```python
from build123d import *

# Parameters (mm, degrees)
F1_DEPTH = 4.4


with BuildPart() as f1:
    # F0 (on Top) → F1 (new body)
    with BuildSketch(Plane.XY):
        with BuildLine():
            ThreePointArc((-12.44334, -91.95904), (-8.617964, -88.425467), (-3.570689, -87.143026))
            Line((-3.570689, -87.143026), (-3.570689, -70.3213))
            Line((-3.570689, -70.3213), (-82.913134, -70.3213))
            Line((-82.913134, -70.3213), (-88.507661, -70.3213))
            Line((-88.507661, -70.3213), (-88.507661, -75.559488))
            Line((-88.507661, -75.559488), (-84.057661, -75.559488))
            Line((-84.057661, -75.559488), (-84.057661, -80.009488))
            Line((-84.057661, -80.009488), (-88.507661, -80.009488))
            Line((-88.507661, -80.009488), (-88.507661, -96.734692))
            ThreePointArc((-88.507661, -96.734692), (-79.443295, -109.014634), (-64.98152, -113.89488))
            Line((-64.98152, -113.89488), (-45.348551, -113.89488))
            ThreePointArc((-45.348551, -113.89488), (-25.575249, -107.908225), (-12.44334, -91.95904))
        make_face()
        with BuildLine():
            ThreePointArc((-78.507661, -78.3213), (-77.628981, -76.199979), (-75.507661, -75.3213))
            Line((-75.507661, -75.3213), (-8.347679, -75.3213))
            ThreePointArc((-8.347679, -75.3213), (-6.986534, -76.530687), (-6.480797, -78.279848))
            Line((-6.480797, -78.279848), (-6.480797, -81.040353))
            Line((-6.480797, -81.040353), (-6.480797, -81.041593))
            ThreePointArc((-6.480797, -81.041593), (-7.309408, -82.599272), (-8.960268, -83.221863))
            ThreePointArc((-8.960268, -83.221863), (-13.595876, -85.631372), (-16.90926, -89.67069))
            ThreePointArc((-16.90926, -89.67069), (-28.184907, -103.637987), (-45.348551, -108.89488))
            Line((-45.348551, -108.89488), (-64.926874, -108.89488))
            ThreePointArc((-64.926874, -108.89488), (-76.195022, -105.191008), (-83.507661, -95.852104))
            Line((-83.507661, -95.852104), (-83.507661, -87.279848))
            ThreePointArc((-83.507661, -87.279848), (-82.921875, -85.865634), (-81.507661, -85.279848))
            ThreePointArc((-81.507661, -85.279848), (-79.386341, -84.401168), (-78.507661, -82.279848))
            Line((-78.507661, -82.279848), (-78.507661, -78.3213))
        make_face(mode=Mode.SUBTRACT)
        with BuildLine():
            Line((80.823653, -96.734275), (80.823653, -85.451687))
            Line((80.823653, -85.451687), (80.823653, -80.451687))
            Line((80.823653, -80.451687), (76.373653, -80.449196))
            Line((76.373653, -80.449196), (76.376145, -75.999196))
            Line((76.376145, -75.999196), (80.823653, -76.001686))
            Line((80.823653, -76.001686), (80.823653, -75.281577))
            Line((80.823653, -75.281577), (80.823653, -70.3213))
            Line((80.823653, -70.3213), (76.384345, -70.3213))
            Line((76.384345, -70.3213), (75.771756, -70.3213))
            Line((75.771756, -70.3213), (-3.570689, -70.3213))
            Line((-3.570689, -70.3213), (-3.570689, -87.143026))
            ThreePointArc((-3.570689, -87.143026), (1.080367, -88.217483), (4.786777, -91.225688))
            ThreePointArc((4.786777, -91.225688), (5.069545, -91.596309), (5.335725, -91.979017))
            ThreePointArc((5.335725, -91.979017), (18.457726, -107.907175), (38.207173, -113.894871))
            ThreePointArc((38.207173, -113.894871), (38.219889, -113.894877), (38.232605, -113.89488))
            Line((38.232605, -113.89488), (57.294375, -113.89488))
            ThreePointArc((57.294375, -113.89488), (71.758098, -109.01535), (80.823653, -96.734275))
        make_face()
        with BuildLine():
            ThreePointArc((9.767882, -89.67069), (9.689205, -89.523601), (9.608648, -89.377533))
            ThreePointArc((9.608648, -89.377533), (6.324286, -85.527112), (1.818889, -83.221863))
            ThreePointArc((1.818889, -83.221863), (0.16803, -82.599272), (-0.660581, -81.041593))
            Line((-0.660581, -81.041593), (-0.660581, -81.040353))
            Line((-0.660581, -81.040353), (-0.660581, -78.279848))
            ThreePointArc((-0.660581, -78.279848), (-0.154844, -76.530687), (1.206301, -75.3213))
            Line((1.206301, -75.3213), (68.366283, -75.3213))
            ThreePointArc((68.366283, -75.3213), (70.487603, -76.199979), (71.366283, -78.3213))
            Line((71.366283, -78.3213), (71.366283, -82.279848))
            ThreePointArc((71.366283, -82.279848), (72.244962, -84.401168), (74.366283, -85.279848))
            ThreePointArc((74.366283, -85.279848), (75.780496, -85.865634), (76.366283, -87.279848))
            Line((76.366283, -87.279848), (76.366283, -95.852104))
            ThreePointArc((76.366283, -95.852104), (69.053644, -105.191008), (57.785496, -108.89488))
            Line((57.785496, -108.89488), (38.207173, -108.89488))
            ThreePointArc((38.207173, -108.89488), (21.043529, -103.637987), (9.767882, -89.67069))
        make_face(mode=Mode.SUBTRACT)
    extrude(amount=F1_DEPTH)


solid = f1.part
```
Check sheet for the modelled part. Datum: model origin and axes. Units: mm. A direction names the side the tool comes from. Coordinates: 2 decimals unless noted, no trailing zeros. Order: outer loops, then holes, each group sorted by start corner. A loop starts at its lowest first (then second) coordinate and runs counter-clockwise, first axis right, second up. Notation, with made-up numbers: M -38.75,-26.5 L -2.75,-26.5 A20 cw -2.75,-2.5 Z; hole C -9,-40 d10. An arc over 180 degrees is marked long. Write each question's results on one line, items separated by ' | '. Start each with the question number.
1. Cross-section at C-C on z = 3.25. State how many separate pieces and enclosed holes the cut face has, and give its area (3 significant figures).
2. Material ranges on probe 1 along Y at (x, z) = (54, 0.65); probe 2 along X at (y, z) = (-87, 2.4); probe 3 along X at (y, z) = (-93, 0.2), recorded low to high.
3. Access from +Z, -Z, +X, -X, +Y, -Y to the whole of each face (thin tool, end or side, straight path). Record for faces 5 (the face through (18.21, -107.74, 2.17)), 6 (the face through (-84.058, -78, 2)), 7 (the face through (34, -75.321, 2)).
4. Cross-section at B-B on y = -99. Record the cut outline in (x, z).
5. Mould release check, pull along Y, two halves, no side actions. Record for faces 1 (the face through (-4, -86, 4.4)), 2 (the face through (48, -113.895, 2)), 3 (the face through (69.191, -105.094, 2.169)), 4 (the face through (-3, -70.321, 2)): +Y half, -Y half, draft (parallel to the pull), parting line (faces both ways), or undercut.
6. Cross-section at A-A on x = -63. Record the cut outline in (y, z).
7. Go/stop test with flat-tipped pins: P1, Ø1.5, axis at y = -107.5, z = 3.5, coming from the +X side; P2, Ø1.2, axis at y = -79.5, z = 2, coming from the +X side; P3, Ø3, axis at x = -15, y = -102, coming from the -Z side; P4, Ø1.3, axis at x = 36.5, z = 3, coming from the -Y side. Record where each tip stops, or that it passes through.
8. Cross-section at D-D on x = 29. Record the cut outline in (y, z).
Checks:
1) separate pieces: 1 | enclosed holes: 2 | area: 2,140 mm²
2) probe 1: y = -113.89 to -108.89, -75.32 to -70.32 | probe 2: x = -88.51 to -83.49, -15.04 to 7.9, 76.35 to 80.82 | probe 3: x = -88.51 to -83.51, -18.49 to -12.9, 5.78 to 11.34, 76.37 to 80.82
3) face 5: +Z, -Z, -Y | face 6: +Z, -Z, -X | face 7: +Z, -Z
4) outline: M -87.61,0 L -81.96,0 L -81.96,4.4 L -87.61,4.4 Z; M -22.8,0 L -16.36,0 L -16.36,4.4 L -22.8,4.4 Z; M 9.25,0 L 15.65,0 L 15.65,4.4 L 9.25,4.4 Z; M 74.82,0 L 79.92,0 L 79.92,4.4 L 74.82,4.4 Z
5) face 1: draft | face 2: -Y half | face 3: undercut | face 4: +Y half
6) outline: M -113.89,0 L -108.89,0 L -108.89,4.4 L -113.89,4.4 Z; M -75.32,0 L -70.32,0 L -70.32,4.4 L -75.32,4.4 Z
7) P1: stops at x = 74.45 | P2: stops at x = 76.37 | P3: passes through | P4: stops at y = -113.88
8) outline: M -112.68,0 L -107.48,0 L -107.48,4.4 L -112.68,4.4 Z; M -75.32,0 L -70.32,0 L -70.32,4.4 L -75.32,4.4 Z
